For this review, take the finished solid that the model builds, in its own axes (mm). Face numbers are marked on the shaded views. A direction names the side the tool comes from. Coordinates: 2 decimals unless noted, no trailing zeros. Loops run counter-clockwise (first coordinate to the right, second up) from the corner with the lowest first, then second, coordinate; pieces in that order, holes last. Notation, with made-up numbers: (9.5, 24) - (30.5, 24) arc R26 cw to (30.5, 59) - close; hole circle Ø3 at (-36, 72.5). An arc over 180 degrees is marked (long way). Answer as a JSON object with one key per item and string values. Group by question number.
Item 1: We need section A-A (z = -4.8). Give the boundary of the cut face in (x, y), then the cut area to 3 significant figures.
Item 2: Mouldability with a two-part tool opening along X and no side actions: class the marked faces 5, 6 and 7 as released by +X, released by -X, zero draft, split by the parting line, or undercut.
Item 3: We need section C-C (y = -15.25). Give the boundary of the cut face in (x, z), then the cut area to 3 significant figures.
Item 4: Tool access review of the marked faces 1, 2, 3 and 4: name each direction out of +Z, -Z, +X, -X, +Y, -Y from which nothing blocks a thin tool from reaching the whole face with its end or side.
Item 5: To check wall thickness, follow line 1 (Y direction, x = 22, z = -12); line 2 (Y direction, x = 15.25, z = -4.8); line 3 (Z direction, x = 8.5, y = -28). State the ranges of each line that lie inside material, in increasing order.
Item 6: Clearance check with flat-ended pins moving along their axes: pin 1 (1.5 mm diameter, centred on x = -5.5, y = -12, fed in from -Z); pin 2 (4 mm diameter, centred on x = 7, y = -5.5, fed in from +Z); pin 3 (5.5 mm diameter, centred on y = -15.5, z = -12.5, fed in from +X); pin 4 (4 mm diameter, centred on y = -2.65, z = -16.07, fed in from -X). State where each tip first meets the part, or that it passes through.
Item 7: We need section D-D (x = -4.5). Give the boundary of the cut face in (y, z), then the cut area to 3 significant figures.
Item 8: We need section B-B (x = 14). Give the boundary of the cut face in (y, z), then the cut area to 3 significant figures.
from build123d import *

# Parameters (mm, degrees)
SKETCH1_W            = 43.35
SKETCH1_H            = 29.15
BOSS_EXTRUDE1_DEPTH  = 30
CUT_EXTRUDE6_DEPTH   = 28.13
SKETCH11_W           = 18.87556933
SKETCH11_H           = 20.106349468
CUT_EXTRUDE8_DEPTH   = 50
SKETCH14_W           = 3
SKETCH14_H           = 29.15
BOSS_EXTRUDE5_DEPTH  = 30
SKETCH15_W           = 8
SKETCH15_H           = 4.023650532
CUT_EXTRUDE10_DEPTH  = 5
SKETCH16_W           = 8
SKETCH16_H           = 4
CUT_EXTRUDE11_DEPTH  = 5
SKETCH17_R           = 1.75
CUT_EXTRUDE12_DEPTH  = 5
CUT_EXTRUDE14_DEPTH  = 50
SKETCH30_R           = 1.25
CUT_EXTRUDE23_DEPTH  = 45
SKETCH31_R           = 1.25
CUT_EXTRUDE24_DEPTH  = 50
SKETCH32_R           = 1.25
CUT_EXTRUDE25_DEPTH  = 50
CUT_EXTRUDE29_DEPTH  = 5
BOSS_EXTRUDE13_DEPTH = 24.1
BOSS_EXTRUDE14_DEPTH = 16.25
SKETCH74_R           = 1.250000003
CUT_EXTRUDE30_DEPTH  = 10


with BuildPart() as part:
    # Sketch1 → Boss-Extrude1 (new body)
    with BuildSketch(Plane.XY):
        with Locations((-32.56399028, -14.719171637)):
            Rectangle(SKETCH1_W, SKETCH1_H)
    extrude(amount=-BOSS_EXTRUDE1_DEPTH)

    # Sketch9 → Cut-Extrude6 (cut)
    with BuildSketch(Plane.XZ.offset(29.294171637)):
        Polygon((-14.88899028, 0), (-18.88899028, -8), (-46.23899028, -8), (-50.23899028, 0), align=None)
    extrude(amount=-CUT_EXTRUDE6_DEPTH, mode=Mode.SUBTRACT)

    # Sketch11 → Cut-Extrude8 (cut)
    with BuildSketch(Plane.ZY.offset(54.23899028)):
        with Locations((-9.437784665, -15.217346371)):
            Rectangle(SKETCH11_W, SKETCH11_H)
    extrude(amount=-CUT_EXTRUDE8_DEPTH, mode=Mode.SUBTRACT)

    # Sketch14 → Boss-Extrude5 (add)
    with BuildSketch(Plane(origin=(0, 0, -30), x_dir=(-1, 0, 0), z_dir=(0, 0, -1))):
        with Locations((36.48899028, -14.719171637)):
            Rectangle(SKETCH14_W, SKETCH14_H)
    extrude(amount=-BOSS_EXTRUDE5_DEPTH)

    # Sketch15 → Cut-Extrude10 (cut)
    with BuildSketch(Plane.ZY.offset(37.98899028)):
        with Locations((-4, -27.282346371)):
            Rectangle(SKETCH15_W, SKETCH15_H)
    extrude(amount=-CUT_EXTRUDE10_DEPTH, mode=Mode.SUBTRACT)

    # Sketch16 → Cut-Extrude11 (cut)
    with BuildSketch(Plane.ZY.offset(37.98899028)):
        with Locations((-4, -3.164171637)):
            Rectangle(SKETCH16_W, SKETCH16_H)
    extrude(amount=-CUT_EXTRUDE11_DEPTH, mode=Mode.SUBTRACT)

    # Sketch17 → Cut-Extrude12 (cut)
    with BuildSketch(Plane.ZY.offset(37.98899028)):
        with Locations((-4.799999988, -19.899171637)):
            Circle(SKETCH17_R)
        with Locations((-4.799999989, -9.549171637)):
            Circle(SKETCH17_R)
    extrude(amount=-CUT_EXTRUDE12_DEPTH, mode=Mode.SUBTRACT)

    # Sketch20 → Cut-Extrude14 (cut)
    with BuildSketch(Plane.ZY.offset(54.23899028)):
        Polygon((-30, -29.294171637), (-30, -0.144171637), (-20.81, -0.144171637), align=None)
    extrude(amount=-CUT_EXTRUDE14_DEPTH, mode=Mode.SUBTRACT)

    # Sketch30 → Cut-Extrude23 (cut)
    with BuildSketch(Plane.ZY.offset(54.23899028)):
        with Locations(Location((-12.001192799, -27.284171637, 0), (0, 0, 270))):
            Circle(SKETCH30_R)
        with Locations(Location((-20.145814089, -27.284171637, 0), (0, 0, 270))):
            Circle(SKETCH30_R)
    extrude(amount=-CUT_EXTRUDE23_DEPTH, mode=Mode.SUBTRACT)

    # Sketch31 → Cut-Extrude24 (cut)
    with BuildSketch(Plane.ZY.offset(54.23899028)):
        with Locations(Location((-16.073503444, -2.654171637, 0), (0, 0, 270))):
            Circle(SKETCH31_R)
    extrude(amount=-CUT_EXTRUDE24_DEPTH, mode=Mode.SUBTRACT)

    # Sketch32 → Cut-Extrude25 (cut)
    with BuildSketch(Plane.ZY.offset(54.23899028)):
        with Locations(Location((-20.609812978, -15.243146641, 0), (0, 0, 270))):
            Circle(SKETCH32_R)
    extrude(amount=-CUT_EXTRUDE25_DEPTH, mode=Mode.SUBTRACT)

    # Sketch56 → Cut-Extrude29 (cut)
    with BuildSketch(Plane.XZ.offset(1.164171637)):
        Polygon((-14.88899028, 0), (-18.88899028, -8), (-46.23899028, -8), (-50.23899028, 0), align=None)
    extrude(amount=-CUT_EXTRUDE29_DEPTH, mode=Mode.SUBTRACT)

    # Sketch68 → Boss-Extrude13 (add)
    with BuildSketch(Plane(origin=(-34.98899028, 0, 0), x_dir=(0, 0, -1), z_dir=(1, 0, 0))):
        Polygon((18.87556933, -5.164171637), (12.53556933, -5.164171637), (18.87556933, -25.270521105), align=None)
    extrude(amount=BOSS_EXTRUDE13_DEPTH)

    # Sketch73 → Boss-Extrude14 (add)
    with BuildSketch(Plane.ZY.offset(37.98899028)):
        Polygon((-18.87556933, -5.164171637), (-12.53556933, -5.164171637), (-18.87556933, -25.270521105), align=None)
    extrude(amount=BOSS_EXTRUDE14_DEPTH)


with BuildPart() as body_2:
    # Mirror1: mirrored copy
    add(part.part.mirror(Plane(origin=(-10.88899028, -0.144171637, -30), x_dir=(0, 0, 1), z_dir=(1, 0, 0))))

    # Sketch74 → Cut-Extrude30 (cut)
    with BuildSketch(Plane(origin=(0, 5.954518238, -18.887291254), x_dir=(-1, 0, 0), z_dir=(0, 0.3006772394057975, -0.953725955242547))):
        with Locations(Location((-19.919214984, -25.5324432, 0), (0, 0, 90))):
            Circle(SKETCH74_R)
        with Locations(Location((-1.538214984, -25.532443188, 0), (0, 0, 90))):
            Circle(SKETCH74_R)
        with Locations(Location((-1.538214991, -14.26893462, 0), (0, 0, 90))):
            Circle(SKETCH74_R)
        with Locations(Location((-19.919214991, -14.268934632, 0), (0, 0, 90))):
            Circle(SKETCH74_R)
    extrude(amount=-CUT_EXTRUDE30_DEPTH, mode=Mode.SUBTRACT)


solid = body_2.part
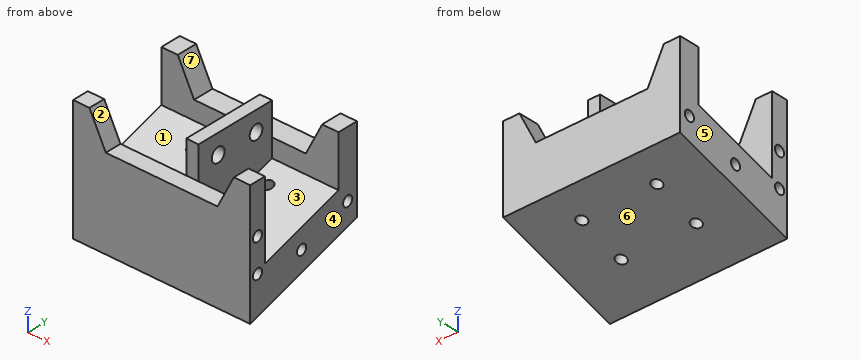
Check sheet entries:
{
 "1": {"outline": "(-10.89, -29.29) - (-4.49, -29.29) - (-4.49, -25.27) - (-10.89, -25.27) - close; (-10.89, -5.16) - (-4.49, -5.16) - (-4.49, -0.14) - (-10.89, -0.14) - close; (13.21, -25.27) - (16.21, -25.27) - (16.21, -21.65) - (13.21, -21.65) - close; (13.21, -18.15) - (16.21, -18.15) - (16.21, -11.3) - (13.21, -11.3) - close; (13.21, -7.8) - (16.21, -7.8) - (16.21, -5.16) - (13.21, -5.16) - close; (26.06, -29.29) - (32.46, -29.29) - (32.46, -25.27) - (26.06, -25.27) - close; (26.06, -5.16) - (32.46, -5.16) - (32.46, -0.14) - (26.06, -0.14) - close", "area": "155 mm2"},
 "2": {"face 5": "released by -X", "face 6": "zero draft", "face 7": "undercut"},
 "3": {"outline": "(-10.89, -25.57) - (32.46, -25.57) - (32.46, -21.86) - (-10.89, -21.86) - close; (-10.89, -19.36) - (32.46, -19.36) - (32.46, -15.72) - (16.21, -15.72) - (16.21, 0) - (13.21, 0) - (13.21, -15.72) - (-10.89, -15.72) - close", "area": "366 mm2"},
 "4": {"face 1": "+Z, -X", "face 2": "+Z, +Y, -Y", "face 3": "+Z, +X", "face 4": "+Z, -Z, +X, +Y, -Y"},
 "5": {"line 1": "y = -29.29 to -28.53, -26.03 to -25.27, -5.16 to -0.14", "line 2": "y = -25.27 to -21.65, -18.15 to -11.3, -7.8 to -5.16", "line 3": "z = -29.59 to -21.17, -19.12 to -13.03, -10.98 to -8"},
 "6": {"pin 1": "stops at z = -24.78", "pin 2": "stops at z = -8", "pin 3": "stops at x = 16.21", "pin 4": "stops at x = -10.89"},
 "7": {"outline": "(-29.29, -30) - (-0.14, -20.81) - (-0.14, -4.78) - (-5.16, -4.78) - (-5.16, -12.54) - (-25.27, -18.88) - (-25.27, -4.78) - (-29.29, -4.78) - close; hole circle Ø2.5 at (-27.28, -20.15); hole circle Ø2.5 at (-27.28, -12); hole circle Ø2.5 at (-15.24, -20.61); hole circle Ø2.5 at (-2.65, -16.07)", "area": "362 mm2"},
 "8": {"outline": "(-29.29, -30) - (-0.14, -20.81) - (-0.14, -8) - (-5.16, -8) - (-5.16, 0) - (-25.27, 0) - (-25.27, -8) - (-29.29, -8) - close; hole circle Ø2.5 at (-27.28, -20.15); hole circle Ø2.5 at (-27.28, -12); hole circle Ø3.5 at (-19.9, -4.8); hole circle Ø2.5 at (-15.24, -20.61); hole circle Ø3.5 at (-9.55, -4.8); hole circle Ø2.5 at (-2.65, -16.07)", "area": "629 mm2"}
}
